```python
from build123d import *

# Parameters (mm, degrees)
BOSS_EXTRUDE1_DEPTH = 12.7
SKETCH3_W           = 27.94
SKETCH3_H           = 15.24
SKETCH3_R           = 1.27
BOSS_EXTRUDE2_DEPTH = 2.54


with BuildPart() as part:
    # Sketch2 → Boss-Extrude1 (new body)
    with BuildSketch(Plane(origin=(0, 0, 0), x_dir=(0, 0, -1), z_dir=(1, 0, 0))):
        Polygon((0, 44.0961272), (-31.75, 44.0961272), (-31.75, -19.4038728), (0, -19.4038728), (0, -13.0538728), (-25.4, -13.0538728), (-25.4, 37.7461272), (0, 37.7461272), align=None)
    extrude(amount=BOSS_EXTRUDE1_DEPTH)

    # Sketch3 → Boss-Extrude2 (add)
    with BuildSketch(Plane(origin=(0, 0, 0), x_dir=(-1, 0, 0), z_dir=(0, 0, -1))):
        with Locations((-6.35, 45.3661272)):
            Rectangle(SKETCH3_W, SKETCH3_H)
        with Locations((-6.35, 48.5411272)):
            Circle(SKETCH3_R, mode=Mode.SUBTRACT)
        with Locations((-6.35, -20.6738728)):
            Rectangle(SKETCH3_W, SKETCH3_H)
        with Locations((-6.35, -23.8488728)):
            Circle(SKETCH3_R, mode=Mode.SUBTRACT)
    extrude(amount=BOSS_EXTRUDE2_DEPTH)


solid = part.part
```
Work out the finished part from the listing and answer in its coordinate system (mm). A direction names the side the tool comes from. Round coordinates to 2 decimals unless told otherwise and drop trailing zeros. Write each loop counter-clockwise with the first axis right and the second up, starting at its lowest first coordinate (ties: lowest second). Pieces come first, ordered by that corner, then holes.
1) Consider probe 1 along Y at (x, z) = (6.35, -1.35); probe 2 along Y at (x, z) = (7, 12.5); probe 3 along X at (y, z) = (20, 28). Determine where each line is inside the solid, lowest interval first.
2) Flat-ended cylindrical pins translate along their axes: P1, Ø3.5, axis at x = 6.35, y = 48.54, coming from the -Z side; P2, Ø10, axis at x = 2, z = 18, coming from the -Y side; P3, Ø9.5, axis at y = 4, z = 23.5, coming from the +X side; P4, Ø16, axis at y = 2, z = 17.5, coming from the -X side. Find the tip coordinate at first contact, or state that the pin passes through.
3) A cutting plane is placed at A-A on x = -3.5. Determine the outline of the cut face in (y, z).
4) A cutting plane is placed at D-D on y = -8.5. Determine the outline of the cut face in (x, z).
5) Which of the six approach directions +Z, -Z, +X, -X, +Y, -Y give full straight-line access (tool end or side, diameter ignored) to faces 1 (the face through (6, 44.096, 16)), 2 (the face through (6, -13.054, 11)), 3 (the face through (6, -19.404, 16)), 4 (the face through (0, 13, 27)), 5 (the face through (6, 13, 31.75))?
6) Determine the mould class of faces 6 (the face through (7, 45, -2.54)), 7 (the face through (7, -28.294, -1)), 8 (the face through (6.625, -25.089, -1.252)) for opening direction Y: pulls with the +Y half, pulls with the -Y half, needs draft (parallel to the pull), parting line crosses it, or undercut.
7) A cutting plane is placed at C-C on x = 6.35. Determine the outline of the cut face in (y, z).
8) A cutting plane is placed at B-B on z = 13.5. Determine the outline of the cut face in (x, y), and give its area (3 significant figures).
Entries:
1. probe 1: y = -28.29 to -25.12, -22.58 to -13.05, 37.75 to 47.27, 49.81 to 52.99
1. probe 2: y = -19.4 to -13.05, 37.75 to 44.1
1. probe 3: x = 0 to 12.7
2. P1: stops at z = -2.54
2. P2: stops at y = -19.4
2. P3: stops at x = 12.7
2. P4: stops at x = 0
3. outline: (-28.29, -2.54) - (-13.05, -2.54) - (-13.05, 0) - (-28.29, 0) - close; (37.75, -2.54) - (52.99, -2.54) - (52.99, 0) - (37.75, 0) - close
4. outline: (0, 25.4) - (12.7, 25.4) - (12.7, 31.75) - (0, 31.75) - close
5. face 1: +Z, +X, -X, +Y
5. face 2: -Z, +X, -X
5. face 3: +Z, +X, -X, -Y
5. face 4: +Z, -X, +Y, -Y
5. face 5: +Z, +X, -X, +Y, -Y
6. face 6: needs draft
6. face 7: pulls with the -Y half
6. face 8: undercut
7. outline: (-28.29, -2.54) - (-25.12, -2.54) - (-25.12, 0) - (-28.29, 0) - close; (-22.58, -2.54) - (-13.05, -2.54) - (-13.05, 25.4) - (37.75, 25.4) - (37.75, -2.54) - (47.27, -2.54) - (47.27, 0) - (44.1, 0) - (44.1, 31.75) - (-19.4, 31.75) - (-19.4, 0) - (-22.58, 0) - close; (49.81, -2.54) - (52.99, -2.54) - (52.99, 0) - (49.81, 0) - close
8. outline: (0, -19.4) - (12.7, -19.4) - (12.7, -13.05) - (0, -13.05) - close; (0, 37.75) - (12.7, 37.75) - (12.7, 44.1) - (0, 44.1) - close
8. area: 161 mm2
